Read the model definition and answer for the solid it produces. Units are mm, in the model's axes. Face numbers are marked on the shaded views. A direction names the side the tool comes from. Coordinates: 2 decimals unless noted, no trailing zeros. Order: outer loops, then holes, each group sorted by start corner. A loop starts at its lowest first (then second) coordinate and runs counter-clockwise, first axis right, second up.
```python
from build123d import *

# Parameters (mm, degrees)
SKETCH1_R           = 27.5
SKETCH1_R_2         = 20
BOSS_EXTRUDE1_DEPTH = 5
SKETCH2_R           = 24
SKETCH2_R_2         = 20
BOSS_EXTRUDE2_DEPTH = 5


with BuildPart() as part:
    # Sketch1 → Boss-Extrude1 (new, symmetric)
    with BuildSketch(Plane.XY):
        Circle(SKETCH1_R)
        Circle(SKETCH1_R_2, mode=Mode.SUBTRACT)
    extrude(amount=BOSS_EXTRUDE1_DEPTH, both=True)

    # Sketch2 → Boss-Extrude2 (add)
    with BuildSketch(Plane.XY.offset(5)):
        Circle(SKETCH2_R)
        Circle(SKETCH2_R_2, mode=Mode.SUBTRACT)
    boss_extrude2 = extrude(amount=BOSS_EXTRUDE2_DEPTH)

    # Mirror1: Boss-Extrude2 across plane
    add(boss_extrude2.mirror(Plane.XY))


solid = part.part
```
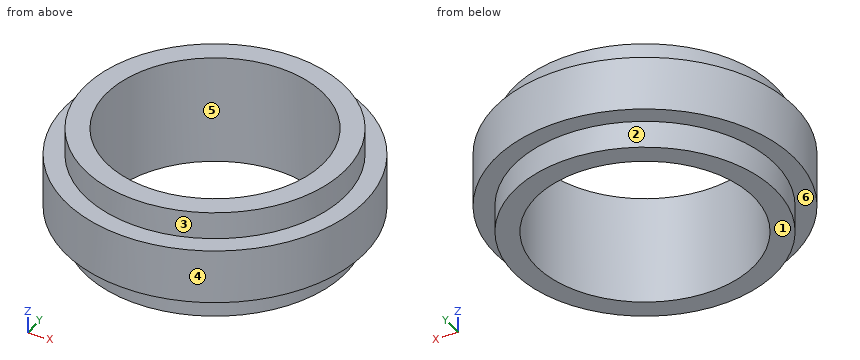
1) A cutting plane is placed at A-A, the plane x = 0. Determine the outline of the cut face in (y, z).
A:
outline: (-27.5, -5) - (-24, -5) - (-24, -10) - (-20, -10) - (-20, 10) - (-24, 10) - (-24, 5) - (-27.5, 5) - close; (20, -10) - (24, -10) - (24, -5) - (27.5, -5) - (27.5, 5) - (24, 5) - (24, 10) - (20, 10) - close
2) Determine the mould class of the marked faces 4, 5 and 6 for opening direction X: pulls with the +X half, pulls with the -X half, needs draft (parallel to the pull), parting line crosses it, or undercut.
A:
face 4: parting line crosses it
face 5: undercut
face 6: needs draft
3) A cutting plane is placed at D-D, the plane z = 3.25. Determine the outline of the cut face in (x, y).
A:
outline: circle Ø55 at (0, 0); hole circle Ø40 at (0, 0)
4) Flat-ended cylindrical pins translate along their axes: pin 1 Ø1.5 at (x, z) = (-5.5, 1) entering from -Y; pin 2 Ø6 at (y, z) = (-10.5, 2) entering from -X; pin 3 Ø12 at (y, z) = (-6.5, 6.5) entering from +X; pin 4 Ø12 at (x, y) = (3.5, 10) entering from +Z. Find the tip coordinate at first contact, or state that the pin passes through.
A:
pin 1: stops at y = -27.09
pin 2: stops at x = -26.46
pin 3: stops at x = 27.49
pin 4: passes through
5) Straight lines are drawn through the part: line 1 (X direction, y = -16.5, z = 8.5); line 2 (X direction, y = 13, z = 1.75); line 3 (Y direction, x = -14.5, z = 3.5). For each, find the intervals that lie inside material, in ascending order.
A:
line 1: x = -17.43 to -11.3, 11.3 to 17.43
line 2: x = -24.23 to -15.2, 15.2 to 24.23
line 3: y = -23.37 to -13.77, 13.77 to 23.37
6) Which of the six approach directions +Z, -Z, +X, -X, +Y, -Y give full straight-line access (tool end or side, diameter ignored) to the marked faces 1, 2 and 3?
A:
face 1: -Z, +X, -X, +Y, -Y
face 2: -Z
face 3: +Z
7) A cutting plane is placed at C-C, the plane z = 7. Determine the outline of the cut face in (x, y), and give its area (3 significant figures).
A:
outline: circle Ø48 at (0, 0); hole circle Ø40 at (0, 0)
area: 553 mm2
